The drawing under review shows one solid part. Ordinate dimensions are in mm from its lowest x, y, z. Give positions to 0.01 mm unless a question says otherwise; leave off trailing zeros. Write each loop counter-clockwise with the first axis right and the second up, starting at its lowest first coordinate (ties: lowest second). Pieces come first, ordered by that corner, then holes.
Q1. We need section A-A (y = 2.5). Write out the cut boundary in (x, z).
Q2. We need section B-B (x = 2.75). Write out the cut boundary in (y, z).
Q3. For line 1 (Y direction, x = 32.75, z = 15.7); line 2 (X direction, y = 30.5, z = 15.55); line 3 (Z direction, x = 28.5, y = 8), list the stretches that pass through material, from the lowest coordinate up.
Q4. We need section D-D (z = 4.75). Write out the cut boundary in (x, y), then the cut area to 3 significant figures.
Q5. Insertion check: P1, Ø1, axis at y = 3.5, z = 17, coming from the -X side; P2, Ø1, axis at x = 21.5, z = 17, coming from the +Y side; P3, Ø4, axis at x = 29.5, y = 4.5, coming from the -Z side. Each pin has a flat end and moves straight along its axis. Give the tip position at first contact, or say it passes through.
Q6. We need section C-C (x = 17). Write out the cut boundary in (y, z), then the cut area to 4 significant figures.
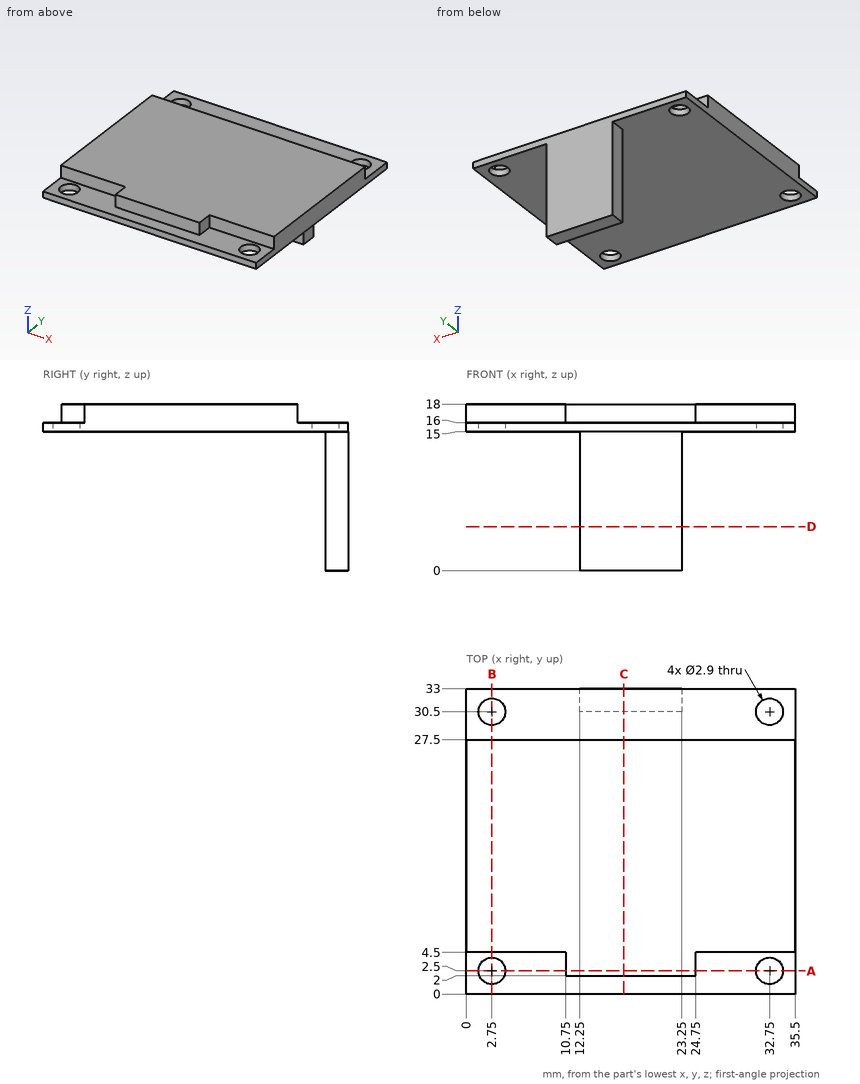
Computed:
1. outline: (0, 15) - (1.3, 15) - (1.3, 16) - (0, 16) - close; (4.2, 15) - (31.3, 15) - (31.3, 16) - (24.75, 16) - (24.75, 18) - (10.75, 18) - (10.75, 16) - (4.2, 16) - close; (34.2, 15) - (35.5, 15) - (35.5, 16) - (34.2, 16) - close
2. outline: (0, 15) - (1.05, 15) - (1.05, 16) - (0, 16) - close; (3.95, 15) - (29.05, 15) - (29.05, 16) - (27.5, 16) - (27.5, 18) - (4.5, 18) - (4.5, 16) - (3.95, 16) - close; (31.95, 15) - (33, 15) - (33, 16) - (31.95, 16) - close
3. line 1: y = 0 to 1.05, 3.95 to 29.05, 31.95 to 33
3. line 2: x = 0 to 1.3, 4.2 to 31.3, 34.2 to 35.5
3. line 3: z = 15 to 18
4. outline: (12.25, 30.5) - (23.25, 30.5) - (23.25, 33) - (12.25, 33) - close
4. area: 27.5 mm2
5. P1: stops at x = 10.75
5. P2: stops at y = 27.5
5. P3: stops at z = 15
6. outline: (0, 15) - (30.5, 15) - (30.5, 0) - (33, 0) - (33, 16) - (27.5, 16) - (27.5, 18) - (2, 18) - (2, 16) - (0, 16) - close
6. area: 121.5 mm2
